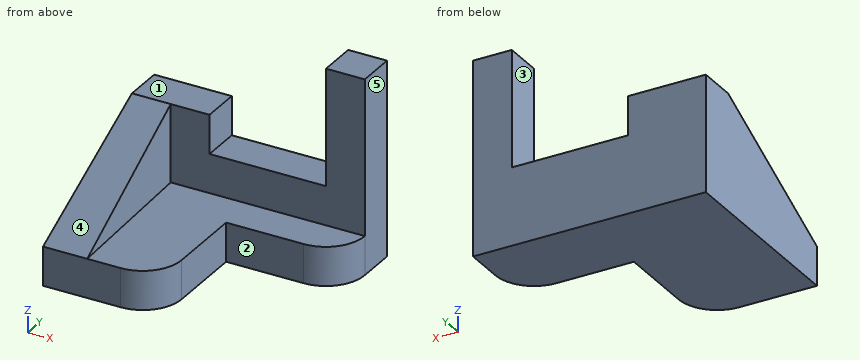
```python
from build123d import *

# Parameters (mm, degrees)
F1_DEPTH  = 10
F2_R      = 10
F3_W      = 10
F3_H      = 10
F4_DEPTH  = 40
F5_W      = 30
F5_H      = 10
F6_DEPTH  = 10
F7_W      = 20
F7_H      = 10
F8_DEPTH  = 20
F10_DEPTH = 20
F11_SIZE2 = 40
F11_SIZE  = 20


with BuildPart() as f1:
    # F0 (on Top) → F1 (new body)
    with BuildSketch(Plane.XY):
        Polygon((60, 0), (0, 0), (0, -50), (30, -50), (30, -20), (60, -20), align=None)
    extrude(amount=F1_DEPTH)

    # F2
    f2_edges = [f1.edges().sort_by_distance(p)[0] for p in [
        (30, -50, 5),
        (60, -20, 5),
    ]]
    fillet(f2_edges, radius=F2_R)

    # F3 (on face) → F4 (join)
    with BuildSketch(Plane.XY.offset(10)):
        with Locations((55, -5)):
            Rectangle(F3_W, F3_H)
    extrude(amount=F4_DEPTH)

    # F5 (on face) → F6 (join)
    with BuildSketch(Plane.XY.offset(10)):
        with Locations((35, -5)):
            Rectangle(F5_W, F5_H)
    extrude(amount=F6_DEPTH)

    # F7 (on face) → F8 (join)
    with BuildSketch(Plane.XY.offset(10)):
        with Locations((10, -5)):
            Rectangle(F7_W, F7_H)
    extrude(amount=F8_DEPTH)

    # F9 (on face) → F10 (join)
    with BuildSketch(Plane.XY.offset(10)):
        Polygon((10, -10), (0, -10), (0, -50), (11.3857937977, -50), align=None)
    extrude(amount=F10_DEPTH)

    # F11
    f11_edges = [f1.edges().sort_by_distance(p)[0] for p in [
        (5.692897, -50, 30),
    ]]
    f11_side = f1.faces().sort_by_distance((7.706899, -50, 12.985998))[0]
    chamfer(f11_edges, length=F11_SIZE, length2=F11_SIZE2, reference=f11_side)


solid = f1.part
```
Build history of the part. All positions in model axes, mm. Face numbers are marked on the shaded views. A direction names the side the tool comes from. Coordinates: 2 decimals unless noted, no trailing zeros. Write each loop counter-clockwise with the first axis right and the second up, starting at its lowest first coordinate (ties: lowest second). Pieces come first, ordered by that corner, then holes.
1. Band-saw the part on C-C, the plane x = 38. Give the cut face in (y, z), and give its area (3 significant figures).
Answer block:
outline: (-20, 0) - (0, 0) - (0, 20) - (-10, 20) - (-10, 10) - (-20, 10) - close
area: 300 mm2
2. Band-saw the part on A-A, the plane z = 25. Give the cut face in (x, y), and give its area (3 significant figures).
Answer block:
outline: (0, -20) - (10.35, -20) - (10, -10) - (20, -10) - (20, 0) - (0, 0) - close; (50, -10) - (60, -10) - (60, 0) - (50, 0) - close
area: 402 mm2
3. Band-saw the part on D-D, the plane z = 34. Give the cut face in (x, y).
Answer block:
outline: (50, -10) - (60, -10) - (60, 0) - (50, 0) - close
4. Band-saw the part on B-B, the plane y = -9. Give the cut face in (x, z).
Answer block:
outline: (0, 0) - (60, 0) - (60, 50) - (50, 50) - (50, 20) - (20, 20) - (20, 30) - (0, 30) - close
5. Drill centre lines: probe 1 along Z at (x, y) = (12, -47); probe 2 along X at (y, z) = (-7, 31.5); probe 3 along Y at (x, z) = (56, 24.5). Where is each one in solid material? Low to high.
Answer block:
probe 1: z = 0 to 10
probe 2: x = 50 to 60
probe 3: y = -10 to 0
6. 3-axis set-ups, long thin cutter, end or side, ignore diameter. For the marked faces 1, 2, 3, 4 and 5: which of +Z, -Z, +X, -X, +Y, -Y reach the whole face in a straight line?
Answer block:
face 1: +Z, -X, +Y, -Y
face 2: +Z, -Z, +X, -Y
face 3: +Z, +Y, -Y
face 4: +Z, +X, -X, -Y
face 5: +Z, -Z, +X, +Y, -Y
7. Drop flat-ended pins along their axis: pin 1 (3 mm diameter, centred on x = 38, z = 7, fed in from -Y); pin 2 (5 mm diameter, centred on y = -37, z = 10, fed in from +X); pin 3 (12 mm diameter, centred on x = 38.5, y = -21.5, fed in from +Z). Give the stop position or say it passes through.
Answer block:
pin 1: stops at y = -20
pin 2: stops at x = 30
pin 3: stops at z = 10
